Here's how the part is built. I have some questions about the finished solid (model axes, mm). Face numbers are marked on the shaded views. A direction names the side the tool comes from. Round coordinates to 2 decimals unless told otherwise and drop trailing zeros. Write each loop counter-clockwise with the first axis right and the second up, starting at its lowest first coordinate (ties: lowest second). Pieces come first, ordered by that corner, then holes. Notation, with made-up numbers: (82, 11) -> (140, 11) arc R22 cw to (140, 46) -> close; hole circle Ø11 at (-6.5, 28.5). An arc over 180 degrees is marked (long way). Answer as CSV lines item,"result".
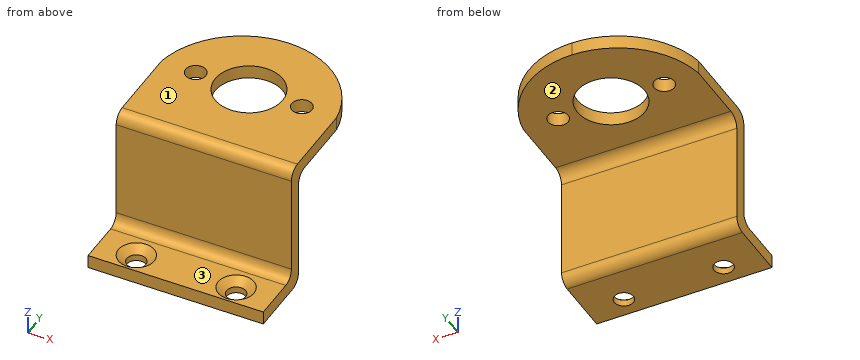
from build123d import *

# Parameters (mm, degrees)
BOSS_EXTRUDE1_DEPTH                       = 41.275
SKETCH3_R                                 = 7.9375
CUT_EXTRUDE2_DEPTH                        = 6.35
SKETCH4_R                                 = 2.38125
CUT_EXTRUDE3_DEPTH                        = 67.959870826
CSK_FOR_8_FLAT_HEAD_MACHINE_SCREW_2_COUNT = 2
CSK_FOR_8_FLAT_HEAD_MACHINE_SCREW_2_PITCH = 23.495


with BuildPart() as part:
    # Sketch1 → Boss-Extrude1 (new body)
    with BuildSketch(Plane(origin=(0, 0, 0), x_dir=(0, 0, -1), z_dir=(1, 0, 0))):
        with BuildLine():
            Line((0, 42.094372261), (0, 9.850328802))
            ThreePointArc((0, 9.850328802), (0.785233991, 7.954606252), (2.680956542, 7.169372261))
            Line((2.680956542, 7.169372261), (26.035, 7.169372261))
            ThreePointArc((26.035, 7.169372261), (27.831051224, 6.425423485), (28.575, 4.629372261))
            Line((28.575, 4.629372261), (28.575, -8.705627739))
            Line((28.575, -8.705627739), (25.4, -8.705627739))
            Line((25.4, -8.705627739), (25.4, 1.454372261))
            ThreePointArc((25.4, 1.454372261), (24.656051224, 3.250423485), (22.86, 3.994372261))
            Line((22.86, 3.994372261), (-0.494043458, 3.994372261))
            ThreePointArc((-0.494043458, 3.994372261), (-2.389766009, 4.779606252), (-3.175, 6.675328802))
            Line((-3.175, 6.675328802), (-3.175, 42.094372261))
            Line((-3.175, 42.094372261), (0, 42.094372261))
        make_face()
    extrude(amount=BOSS_EXTRUDE1_DEPTH)

    # Sketch3 → Cut-Extrude2 (cut)
    with BuildSketch(Plane.XY.offset(3.175)):
        with Locations((20.6375, 24.384850532)):
            Circle(SKETCH3_R)
    extrude(amount=-CUT_EXTRUDE2_DEPTH, mode=Mode.SUBTRACT)

    # Sketch4 → Cut-Extrude3 (cut, through all)
    with BuildSketch(Plane.XY.offset(3.175)):
        with BuildLine():
            Line((0, 42.094372261), (0, 24.384850532))
            ThreePointArc((0, 24.384850532), (7.04031678, 37.060079652), (20.6375, 42.094372261))
            Line((20.6375, 42.094372261), (0, 42.094372261))
        make_face()
        with BuildLine():
            Line((41.275, 42.094372261), (20.6375, 42.094372261))
            ThreePointArc((20.6375, 42.094372261), (34.23468322, 37.060079652), (41.275, 24.384850532))
            Line((41.275, 24.384850532), (41.275, 42.094372261))
        make_face()
        with Locations((8.14050126, 24.314372261)):
            Circle(SKETCH4_R)
        with Locations((33.13410126, 24.314372261)):
            Circle(SKETCH4_R)
    extrude(amount=-CUT_EXTRUDE3_DEPTH, mode=Mode.SUBTRACT)

    # Sketch10 → CSK for #8 Flat Head Machine Screw (100)2 (revolve, cut)
    with BuildSketch(Plane(origin=(8.89, -3.943127739, -25.4), x_dir=(0, -1, 0), z_dir=(1, 0, 0))):
        Polygon((0, 0), (0, 3.175), (2.2479, 3.175), (2.2479, 1.651767624), (4.2164, 0), align=None)
    csk_for_8_flat_head_machine_screw_100 = revolve(axis=Axis((8.89, -3.943127739, -19.05), (0, 0, -1)), mode=Mode.SUBTRACT)

    # CSK for _8 Flat Head Machine Screw _ 2: CSK for #8 Flat Head Machine Screw (100)2 ×2
    with Locations(*[(i * CSK_FOR_8_FLAT_HEAD_MACHINE_SCREW_2_PITCH, 0, 0) for i in range(1, CSK_FOR_8_FLAT_HEAD_MACHINE_SCREW_2_COUNT)]):
        add(csk_for_8_flat_head_machine_screw_100, mode=Mode.SUBTRACT)


solid = part.part
Item 1: For the marked faces 1, 2 and 3, which set-ups out of +Z, -Z, +X, -X, +Y, -Y let a thin tool reach every point of the face, with its end or its side?
Results found:
face 1,"+Z, +X, -X, +Y, -Y"
face 2,"-Z, +X, -X, +Y"
face 3,"+Z, +X, -X, -Y"
Item 2: I need wall thicknesses on L1, parallel to Y at x = 15, z = -3; L2, parallel to Z at x = 36.5, y = 26.5 (3 decimals); L3, parallel to Y at x = 8, z = -27. Which ranges of each line are inside material? Lowest first, please.
Results found:
L1,"y = 3.99 to 7.17"
L2,"z = 0 to 3.175"
L3,"y = -8.71 to -6.07, -1.81 to 6.98"
Item 3: Suppose I cut it at D-D, the plane z = -10. List the corners of the cut face in (x, y) for me (3 decimals), then the cut area to 3 significant figures.
Results found:
outline,"(0, 3.994) -> (41.275, 3.994) -> (41.275, 7.169) -> (0, 7.169) -> close"
area,"131 mm²"
Item 4: Will these pins go through, and if not, where does the flat tip stop? pin 1 (1.5 mm diameter, centred on x = 6.5, y = 15.5, fed in from -Z); pin 2 (11.5 mm diameter, centred on x = 29, z = -8, fed in from -Y); pin 3 (11.5 mm diameter, centred on x = 22.5, z = -9, fed in from +Y).
Results found:
pin 1,"stops at z = 0"
pin 2,"stops at y = 3.99"
pin 3,"stops at y = 7.17"
Item 5: Suppose I cut it at A-A, the plane y = 18.5. List the corners of the cut face in (x, z) for me (3 decimals).
Results found:
outline,"(0, 0) -> (15.311, 0) -> (15.311, 3.175) -> (0, 3.175) -> close; (25.964, 0) -> (41.275, 0) -> (41.275, 3.175) -> (25.964, 3.175) -> close"
Item 6: Suppose I cut it at C-C, the plane x = 19.5. List the corners of the cut face in (y, z) for me (3 decimals), then the cut area to 3 significant figures.
Results found:
outline,"(-8.706, -28.575) -> (4.629, -28.575) arc R2.54 ccw to (7.169, -26.035) -> (7.169, -2.681) arc R2.681 cw to (9.85, 0) -> (16.529, 0) -> (16.529, 3.175) -> (6.675, 3.175) arc R2.681 ccw to (3.994, 0.494) -> (3.994, -22.86) arc R2.54 cw to (1.454, -25.4) -> (-8.706, -25.4) -> close; (32.24, 0) -> (42.063, 0) -> (42.063, 3.175) -> (32.24, 3.175) -> close"
area,"202 mm²"
Item 7: Suppose I cut it at B-B, the plane x = 8.89. List the corners of the cut face in (y, z) for me (3 decimals), then the cut area to 3 significant figures.
Results found:
outline,"(-8.706, -28.575) -> (-6.191, -28.575) -> (-6.191, -27.052) -> (-8.16, -25.4) -> (-8.706, -25.4) -> close; (-1.695, -28.575) -> (4.629, -28.575) arc R2.54 ccw to (7.169, -26.035) -> (7.169, -2.681) arc R2.681 cw to (9.85, 0) -> (22.054, 0) -> (22.054, 3.175) -> (6.675, 3.175) arc R2.681 ccw to (3.994, 0.494) -> (3.994, -22.86) arc R2.54 cw to (1.454, -25.4) -> (0.273, -25.4) -> (-1.695, -27.052) -> close; (26.575, 0) -> (38.476, 0) -> (38.476, 3.175) -> (26.575, 3.175) -> close"
area,"209 mm²"
